Could you check a few things on this model? Use its own coordinates, in mm. A direction names the side the tool comes from. Give positions to 0.01 mm unless a question says otherwise; leave off trailing zeros. Write each loop counter-clockwise with the first axis right and the second up, starting at its lowest first coordinate (ties: lowest second). Pieces come first, ordered by that corner, then holes. Notation, with made-up numbers: (-21, 8.25) - (-7, 8.25) arc R27 cw to (-7, 33.25) - close; hole circle Ø3 at (-30, 6.5). An arc over 180 degrees is marked (long way). Answer as CSV lines item,"result". Start each with the question number.
Q1. Imagine slicing it at A-A on x = 238. List the corners of the cut face in (y, z) for me, and give its area (3 significant figures).
Q2. Will these pins go through, and if not, where does the flat tip stop? pin 1 Ø12.5 at (y, z) = (-13, 1.5) entering from -X; pin 2 Ø5 at (y, z) = (-21, -34) entering from +X; pin 3 Ø7.5 at (y, z) = (-14.5, 1) entering from +X; pin 4 Ø4 at (x, z) = (95, -23) entering from -Y.
Q3. Imagine slicing it at D-D on y = -21.25. State how many separate pieces and enclosed holes the cut face has, and give its area (3 significant figures).
Q4. We'd pull the mould along X, two halves only. Please class faces 6 (the face through (-139, -13, 50.8)), 7 (the face through (-295.299, -12.522, 39.935)), 8 (the face through (12.7, -13, -38)): pulls with the +X half, pulls with the -X half, needs draft (parallel to the pull), parting line crosses it, or undercut.
Q5. If I drill on line 1 along X through (y, z) = (-22.25, 7); line 2 along Z through (x, y) = (240, -12.25); line 3 along X through (y, z) = (-7.5, 23.5), over which ranges is the centre line in solid material (lowest first)?
Q6. On a 3-axis mill with a long thin cutter (end or side, diameter ignored), from which of +Z, -Z, +X, -X, +Y, -Y can I reach the whole of each face in a straight line? I mean faces 1 (the face through (294, -13, -12.7)), 2 (the face through (0, -13, -25.4)), 3 (the face through (-294, -13, 12.7)), 4 (the face through (255.956, -13, 0)), 5 (the face through (-4, 0, 1)). Say none if no direction works.
Q7. Imagine slicing it at C-C on z = -38. List the corners of the cut face in (x, y) for me.
Q8. Imagine slicing it at B-B on z = -7. List the corners of the cut face in (x, y) for me.
```python
from build123d import *

# Parameters (mm, degrees)
F1_DEPTH = 25.4
F2_W     = 25.4
F2_H     = 25.4
F3_DEPTH = 25.4


with BuildPart() as f1:
    # F0 (on Front) → F1 (new body)
    with BuildSketch(Plane.XZ):
        with BuildLine():
            Line((-306.7558, 12.7), (-281.3558, 12.7))
            Line((-281.3558, 12.7), (-281.3558, -12.7))
            Line((-281.3558, -12.7), (-306.7558, -12.7))
            ThreePointArc((-306.7558, -12.7), (-295.596568, -39.640768), (-268.6558, -50.8))
            Line((-268.6558, -50.8), (0, -50.8))
            Line((0, -50.8), (268.6558, -50.8))
            ThreePointArc((268.6558, -50.8), (295.596568, -39.640768), (306.7558, -12.7))
            Line((306.7558, -12.7), (281.3558, -12.7))
            Line((281.3558, -12.7), (281.3558, 12.7))
            Line((281.3558, 12.7), (306.7558, 12.7))
            ThreePointArc((306.7558, 12.7), (295.596568, 39.640768), (268.6558, 50.8))
            Line((268.6558, 50.8), (0, 50.8))
            Line((0, 50.8), (-268.6558, 50.8))
            ThreePointArc((-268.6558, 50.8), (-295.596568, 39.640768), (-306.7558, 12.7))
        make_face()
        with BuildLine():
            Line((-38.1, -25.4), (-243.2558, -25.4))
            ThreePointArc((-243.2558, -25.4), (-252.236056, -21.680256), (-255.9558, -12.7))
            Line((-255.9558, -12.7), (-255.9558, 12.7))
            ThreePointArc((-255.9558, 12.7), (-252.236056, 21.680256), (-243.2558, 25.4))
            Line((-243.2558, 25.4), (-38.1, 25.4))
            ThreePointArc((-38.1, 25.4), (-29.119744, 21.680256), (-25.4, 12.7))
            Line((-25.4, 12.7), (-25.4, -12.7))
            ThreePointArc((-25.4, -12.7), (-29.119744, -21.680256), (-38.1, -25.4))
        make_face(mode=Mode.SUBTRACT)
        with BuildLine():
            ThreePointArc((255.9558, -12.7), (252.236056, -21.680256), (243.2558, -25.4))
            Line((243.2558, -25.4), (38.1, -25.4))
            ThreePointArc((38.1, -25.4), (29.119744, -21.680256), (25.4, -12.7))
            Line((25.4, -12.7), (25.4, 12.7))
            ThreePointArc((25.4, 12.7), (29.119744, 21.680256), (38.1, 25.4))
            Line((38.1, 25.4), (243.2558, 25.4))
            ThreePointArc((243.2558, 25.4), (252.236056, 21.680256), (255.9558, 12.7))
            Line((255.9558, 12.7), (255.9558, -12.7))
        make_face(mode=Mode.SUBTRACT)
    extrude(amount=F1_DEPTH)

    # F2 (on face) → F3 (cut)
    with BuildSketch(Plane.XZ.offset(25.4)):
        with Locations((0, 38.1)):
            Rectangle(F2_W, F2_H)
        with Locations((0, -38.1)):
            Rectangle(F2_W, F2_H)
    extrude(amount=-F3_DEPTH, mode=Mode.SUBTRACT)


solid = f1.part
```
Conclusion:
1,outline,"(-25.4, -50.8) - (0, -50.8) - (0, -25.4) - (-25.4, -25.4) - close; (-25.4, 25.4) - (0, 25.4) - (0, 50.8) - (-25.4, 50.8) - close"
1,area,"1,290 mm^2"
2,pin 1,"x = -281.36"
2,pin 2,"x = 301.79"
2,pin 3,"x = 281.36"
2,pin 4,"through"
3,separate pieces,"1"
3,enclosed holes,"2"
3,area,"35,400 mm^2"
4,face 6,"needs draft"
4,face 7,"pulls with the -X half"
4,face 8,"undercut"
5,line 1,"-281.36 to -255.96, -25.4 to 25.4, 255.96 to 281.36"
5,line 2,"-50.8 to -25.4, 25.4 to 50.8"
5,line 3,"-305.19 to -249.94, -31.42 to 31.42, 249.94 to 305.19"
6,face 1,"+X, +Y, -Y"
6,face 2,"-Z, +Y, -Y"
6,face 3,"-X, +Y, -Y"
6,face 4,"+Y, -Y"
6,face 5,"+Z, -Z, +X, -X, +Y"
7,outline,"(-297.14, -25.4) - (-12.7, -25.4) - (-12.7, 0) - (-297.14, 0) - close; (12.7, -25.4) - (297.14, -25.4) - (297.14, 0) - (12.7, 0) - close"
8,outline,"(-281.36, -25.4) - (-255.96, -25.4) - (-255.96, 0) - (-281.36, 0) - close; (-25.4, -25.4) - (25.4, -25.4) - (25.4, 0) - (-25.4, 0) - close; (255.96, -25.4) - (281.36, -25.4) - (281.36, 0) - (255.96, 0) - close"
